```python
from build123d import *

# Parameters (mm, degrees)
SKETCH1_W           = 5
SKETCH1_H           = 30
BOSS_EXTRUDE1_DEPTH = 100
SKETCH4_R           = 9
SKETCH4_R_2         = 1.5
CUT_EXTRUDE2_DEPTH  = 10


with BuildPart() as part:
    # Sketch1 → Boss-Extrude1 (new, symmetric)
    with BuildSketch(Plane(origin=(0, 0, 0), x_dir=(0, 0, -1), z_dir=(1, 0, 0))):
        with Locations((2.5, 15)):
            Rectangle(SKETCH1_W, SKETCH1_H)
    extrude(amount=BOSS_EXTRUDE1_DEPTH, both=True)

    # Sketch4 → Cut-Extrude2 (cut)
    with BuildSketch(Plane.XY):
        with Locations((0, 15)):
            Circle(SKETCH4_R)
        with Locations((60, 15)):
            Circle(SKETCH4_R)
        with Locations((-60, 15)):
            Circle(SKETCH4_R)
        with Locations((-95, 5)):
            Circle(SKETCH4_R_2)
        with Locations((95, 5)):
            Circle(SKETCH4_R_2)
    extrude(amount=-CUT_EXTRUDE2_DEPTH, mode=Mode.SUBTRACT)


solid = part.part
```
CAD build for the part. Positions are in the model's coordinates, mm. Round coordinates to 2 decimals unless told otherwise and drop trailing zeros. Loops run counter-clockwise (first coordinate to the right, second up) from the corner with the lowest first, then second, coordinate; pieces in that order, holes last. Notation, with made-up numbers: (-29.5, 74.5) - (22.5, 74.5) arc R29 ccw to (22.5, 97.5) - close; hole circle Ø2 at (-15.75, 72). An arc over 180 degrees is marked (long way). Return JSON: item names as keys, results as strings. Group by question number.
Q1. Band-saw the part on B-B on z = -0.8. Give the cut face in (x, y).
Q2. Band-saw the part on A-A on y = 15. Give the cut face in (x, z).
Q3. Two-plate mould, pull along Y, no slides. Class faces 1 (the face through (68.584, 17.703, -2.465)), 2 (the face through (1, 5, 0)), 3 (the face through (1, 0, -2)): +Y half, -Y half, draft (parallel to the pull), parting line (faces both ways), or undercut.
Q4. Drill centre lines: line 1 along Y through (x, z) = (0, -3.25); line 2 along X through (y, z) = (9.75, -2.65); line 3 along Y through (x, z) = (-95, -1.65). Where is each one in solid material? Low to high. Write a range as [from, to].
Q5. Band-saw the part on C-C on x = 0. Give the cut face in (y, z), plus the area to 3 significant figures.
Q6. Flat gauge pin, fed straight in: pin 1 Ø2.5 at (x, y) = (95, 5) entering from -Z. Where does the tip first touch, or does it go through?
Solutions:
{
 "1": {"outline": "(-100, 0) - (100, 0) - (100, 30) - (-100, 30) - close; hole circle Ø3 at (-95, 5); hole circle Ø18 at (-60, 15); hole circle Ø18 at (0, 15); hole circle Ø18 at (60, 15); hole circle Ø3 at (95, 5)"},
 "2": {"outline": "(-100, -5) - (-69, -5) - (-69, 0) - (-100, 0) - close; (-51, -5) - (-9, -5) - (-9, 0) - (-51, 0) - close; (9, -5) - (51, -5) - (51, 0) - (9, 0) - close; (69, -5) - (100, -5) - (100, 0) - (69, 0) - close"},
 "3": {"face 1": "undercut", "face 2": "draft", "face 3": "-Y half"},
 "4": {"line 1": "y = [0, 6], [24, 30]", "line 2": "x = [-100, -67.31], [-52.69, -7.31], [7.31, 52.69], [67.31, 100]", "line 3": "y = [0, 3.5], [6.5, 30]"},
 "5": {"outline": "(0, -5) - (6, -5) - (6, 0) - (0, 0) - close; (24, -5) - (30, -5) - (30, 0) - (24, 0) - close", "area": "60.0 mm^2"},
 "6": {"pin 1": "passes through"}
}
